The model under review builds one solid part; all positions refer to its coordinate system, in mm. Face numbers are marked on the shaded views. A direction names the side the tool comes from. Round coordinates to 2 decimals unless told otherwise and drop trailing zeros. Write each loop counter-clockwise with the first axis right and the second up, starting at its lowest first coordinate (ties: lowest second). Pieces come first, ordered by that corner, then holes. Notation, with made-up numbers: (60, -1) - (83, -1) arc R30 ccw to (83, 32) - close; hole circle Ø5 at (77, 35.5). An arc over 180 degrees is marked (long way). Return JSON: item names as keys, results as strings.
from build123d import *

# Parameters (mm, degrees)
F0_R     = 12.5
F1_DEPTH = 20
F3_R     = 12.5
F4_DEPTH = 10
F5_W     = 18.4501476586
F5_H     = 50
F6_DEPTH = 20
F7_R     = 5
F8_W     = 14.6253928542
F8_H     = 7.4752001092
F8_W_2   = 16.5754444897
F8_H_2   = 11.7003135383
F9_DEPTH = 50.001


with BuildPart() as f1:
    # F0 (on Front) → F1 (new body)
    with BuildSketch(Plane.XZ):
        with BuildLine():
            Line((-50, -25), (0, -25))
            ThreePointArc((0, -25), (25, 0), (0, 25))
            Line((0, 25), (-50, 25))
            Line((-50, 25), (-50, -25))
        make_face()
        Circle(F0_R, mode=Mode.SUBTRACT)
    extrude(amount=F1_DEPTH)



with BuildPart() as f4:
    # F3 (on offset) → F4 (new body)
    with BuildSketch(Plane.XZ.offset(40)):
        with BuildLine():
            Line((-50, 25), (-50, -25))
            Line((-50, -25), (0, -25))
            ThreePointArc((0, -25), (25, 0), (0, 25))
            Line((0, 25), (-50, 25))
        make_face()
        Circle(F3_R, mode=Mode.SUBTRACT)
    extrude(amount=F4_DEPTH)


with BuildPart() as f1_1:
    add(f1.part)

    add(f4.part)  # F6 merges F4
    # F5 (on face) → F6 (join, through all)
    with BuildSketch(Plane.XZ.offset(20)):
        with Locations((-40.7749261707, 0)):
            Rectangle(F5_W, F5_H)
    extrude(amount=F6_DEPTH)

    # F7
    f7_edges = [f1_1.edges().sort_by_distance(p)[0] for p in [
        (-25, -50, 25),
        (-50, -50, 0),
        (-25, -50, -25),
        (25, -50, 0),
        (-12.5, -50, 0),
    ]]
    fillet(f7_edges, radius=F7_R)

    # F8 (on face) → F9 (cut, through all)
    with BuildSketch(Plane.XZ.offset(50)):
        with Locations((-29.1888378561, 9.4781569205)):
            Rectangle(F8_W, F8_H)
        with Locations((-30.9763848782, -8.2348193973)):
            Rectangle(F8_W_2, F8_H_2)
    extrude(amount=-F9_DEPTH, mode=Mode.SUBTRACT)


solid = f1_1.part
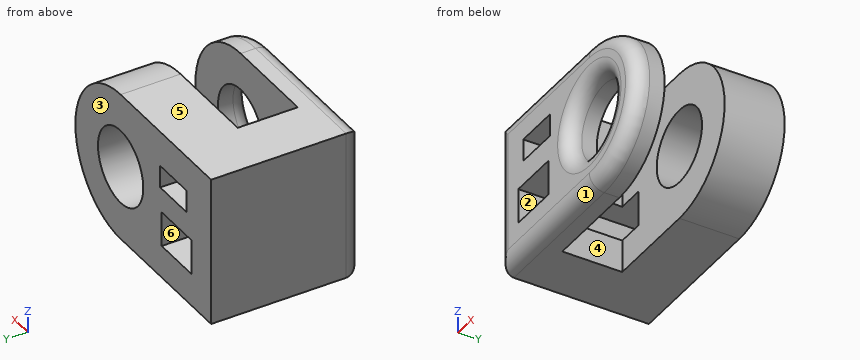
(1) For the marked faces 4, 5 and 6, list the 3-axis set-ups (+Z, -Z, +X, -X, +Y, -Y) from which the entire face can be reached by the end or side of a thin tool; tool diameter is ignored.
Filled in:
{"face 4": "+Z, -Z, +X", "face 5": "+Z, +X, -X, +Y, -Y", "face 6": "+Y, -Y"}
(2) Wall thickness on line 1 (Z direction, x = -28.5, y = -19); line 2 (Y direction, x = -31, z = 14); line 3 (Z direction, x = 0, y = -41.95): over which ranges is each line inside the solid? List them lowest first.
Filled in:
{"line 1": "z = -25 to -14.08, -2.38 to 5.74, 13.22 to 25", "line 2": "y = -50 to -40, -20 to 0", "line 3": "z = -25 to -12.5, 12.5 to 25"}
(3) Clearance check with flat-ended pins moving along their axes: pin 1 Ø6 at (y, z) = (-30.5, -7) entering from +X; pin 2 Ø4 at (y, z) = (-27, 0.5) entering from +X. State where each tip first meets the part, or that it passes through.
Filled in:
{"pin 1": "stops at x = -39.26", "pin 2": "stops at x = -31.55"}
(4) Mouldability with a two-part tool opening along Z and no side actions: class the marked faces 1, 2 and 3 as released by +Z, released by -Z, zero draft, split by the parting line, or undercut.
Filled in:
{"face 1": "released by -Z", "face 2": "undercut", "face 3": "zero draft"}
(5) Add section B-B (z = 0). Write out the cut boundary in (x, y).
Filled in:
{"outline": "(-50, -45) arc R5 ccw to (-45, -50) - (-17.5, -50) arc R5 ccw to (-12.5, -45) - (-12.5, -40) - (-31.55, -40) - (-31.55, -20) - (-12.5, -20) - (-12.5, 0) - (-50, 0) - close; (12.5, -45) arc R5 ccw to (17.5, -50) - (20, -50) arc R5 ccw to (25, -45) - (25, -40) - (12.5, -40) - close; (12.5, -20) - (25, -20) - (25, 0) - (12.5, 0) - close"}
(6) Add section D-D (y = -23.5). Write out the cut boundary in (x, z).
Filled in:
{"outline": "(-50, -25) - (-31.55, -25) - (-31.55, -14.08) - (-39.26, -14.08) - (-39.26, -2.38) - (-31.55, -2.38) - (-31.55, 5.74) - (-36.5, 5.74) - (-36.5, 13.22) - (-31.55, 13.22) - (-31.55, 25) - (-50, 25) - close"}
(7) Add section A-A (y = -6.5). Write out the cut boundary in (x, z).
Filled in:
{"outline": "(-50, -25) - (0, -25) arc R25 ccw to (0, 25) - (-50, 25) - close; hole (-39.26, -14.08) - (-22.69, -14.08) - (-22.69, -2.38) - (-39.26, -2.38) - close; hole (-36.5, 5.74) - (-21.88, 5.74) - (-21.88, 13.22) - (-36.5, 13.22) - close; hole circle Ø25 at (0, 0)"}
(8) Add section C-C (x = -21). Write out the cut boundary in (y, z).
Filled in:
{"outline": "(-50, -20) arc R5 ccw to (-45, -25) - (-40, -25) - (-40, 25) - (-45, 25) arc R5 ccw to (-50, 20) - close; (-20, -25) - (0, -25) - (0, 25) - (-20, 25) - close"}
